The listing builds one solid part. Answer for the finished solid, in the listing's coordinates (mm). Coordinates: 2 decimals unless noted, no trailing zeros. Order: outer loops, then holes, each group sorted by start corner. A loop starts at its lowest first (then second) coordinate and runs counter-clockwise, first axis right, second up. Notation, with made-up numbers: (79, 17) -> (119, 17) arc R26 cw to (119, 39) -> close; hole circle Ø6 at (26, 6). An arc over 180 degrees is marked (long way). Return JSON: item names as keys, results as strings.
```python
from build123d import *

# Parameters (mm, degrees)
SKETCH1_R          = 3
EXTRUDE1_DEPTH     = 260
SKETCH2_R          = 1.25
CUT_EXTRUDE1_DEPTH = 20
CUT_EXTRUDE2_START = -20
SKETCH3_R          = 1.25
CUT_EXTRUDE2_DEPTH = 20
FILLET1_R          = 0.1


with BuildPart() as part:
    # Sketch1 → Extrude1 (new body)
    with BuildSketch(Plane.XY):
        Circle(SKETCH1_R)
    extrude(amount=EXTRUDE1_DEPTH)

    # Sketch2 → Cut-Extrude1 (cut)
    with BuildSketch(Plane.XY.offset(260)):
        Circle(SKETCH2_R)
    extrude(amount=-CUT_EXTRUDE1_DEPTH, mode=Mode.SUBTRACT)

    # Sketch3 → Cut-Extrude2 (cut)
    with BuildSketch(Plane(origin=(0, 0, 0), x_dir=(-1, 0, 0), z_dir=(0, 0, -1)).offset(CUT_EXTRUDE2_START)):
        with Locations(Location((0, 0, 0), (0, 0, 180))):
            Circle(SKETCH3_R)
    extrude(amount=CUT_EXTRUDE2_DEPTH, mode=Mode.SUBTRACT)

    # Fillet1
    fillet1_edges = [part.edges().sort_by_distance(p)[0] for p in [
        (-1.25, 0, 0),
        (-3, 0, 0),
        (-3, 0, 260),
        (-1.25, 0, 260),
    ]]
    fillet(fillet1_edges, radius=FILLET1_R)


solid = part.part
```
Item 1: Find the intervals of material crossed by probe 1 along Y at (x, z) = (0, 14); probe 2 along Z at (x, y) = (2.5, 1.5); probe 3 along Z at (x, y) = (0.5, 0.5), in increasing order.
Answer list:
{"probe 1": "-3 to -1.25, 1.25 to 3", "probe 2": "0 to 260", "probe 3": "20 to 240"}
Item 2: The part is cut by section A-A on y = 0. Determine the outline of the cut face in (x, z).
Answer list:
{"outline": "(-3, 0.1) arc R0.1 ccw to (-2.9, 0) -> (-1.35, 0) arc R0.1 ccw to (-1.25, 0.1) -> (-1.25, 20) -> (1.25, 20) -> (1.25, 0.1) arc R0.1 ccw to (1.35, 0) -> (2.9, 0) arc R0.1 ccw to (3, 0.1) -> (3, 259.9) arc R0.1 ccw to (2.9, 260) -> (1.35, 260) arc R0.1 ccw to (1.25, 259.9) -> (1.25, 240) -> (-1.25, 240) -> (-1.25, 259.9) arc R0.1 ccw to (-1.35, 260) -> (-2.9, 260) arc R0.1 ccw to (-3, 259.9) -> close"}
Item 3: Flat-ended cylindrical pins translate along their axes: pin 1 (1 mm diameter, centred on x = 2, z = 159, fed in from +Y); pin 2 (2 mm diameter, centred on x = 0, y = 0, fed in from -Z); pin 3 (2 mm diameter, centred on x = 0, y = 0, fed in from +Z). Find the tip coordinate at first contact, or state that the pin passes through.
Answer list:
{"pin 1": "y = 2.6", "pin 2": "z = 20", "pin 3": "z = 240"}
Item 4: The part is cut by section C-C on z = 230. Determine the outline of the cut face in (x, y).
Answer list:
{"outline": "circle Ø6 at (0, 0)"}
